Work out the finished part from the listing and answer in its coordinate system (mm). A direction names the side the tool comes from. Coordinates: 2 decimals unless noted, no trailing zeros. Write each loop counter-clockwise with the first axis right and the second up, starting at its lowest first coordinate (ties: lowest second). Pieces come first, ordered by that corner, then holes. Notation, with made-up numbers: (-23, 28.5) - (-16, 28.5) arc R20 ccw to (-16, 64.5) - close; hole circle Ø11 at (-4.75, 70). An arc over 180 degrees is marked (long way). Use a Markdown table: item, result. Add a question column.
(1) Given pin 1 Ø3 at (x, y) = (-41, 30) entering from +Z; pin 2 Ø5 at (x, z) = (-51.5, -6) entering from -Y; pin 3 Ø17 at (x, y) = (-66, 11.5) entering from +Z, each flat-ended and moving along its own axis, determine where each tip first touches the part or whether it passes through.
(2) For a pull along X with two mould halves and no side action, classify faces 5 (the face through (-78, 62, -127)), 6 (the face through (1, 0, 1)), 7 (the face through (54.98, 46.16, -63.82)) as released by +X, released by -X, zero draft, split by the parting line, or undercut.
(3) The part is cut by section A-A, the plane y = 49.5. Give the vertices of the cut face in (x, z), then the cut area to 3 significant figures.
(4) The part is cut by section C-C, the plane z = 97.5. Give the vertices of the cut face in (x, y), then the cut area to 3 significant figures.
(5) The part is cut by section B-B, the plane y = 70.5. Give the vertices of the cut face in (x, z), then the cut area to 4 significant figures.
(6) Find the intervals of material crossed by line 1 (X direction, y = 47, z = 97); line 2 (Z direction, x = 20.5, y = 42); line 3 (Z direction, x = -20, y = 42.5), in increasing order. Write a range as from..to.
(7) A tool of negligible diameter and unlimited length cuts with its end or side. For faces 1 (the face through (-68, 20, -47.5)), 2 (the face through (-29.53, 19.76, 50.84)), 3 (the face through (54.98, 46.16, 131.18)), 4 (the face through (29.041, 19.762, 51.032)), from which of +Z, -Z, +X, -X, +Y, -Y can it reach the whole face along a straight path? Write none if from no direction.
(8) The part is cut by section D-D, the plane x = 56.5. Give the vertices of the cut face in (y, z), then the cut area to 3 significant figures.
Autodesk Inventor part; units mm, degrees
ref_plane "YZ Plane" through (0, 0, 0) normal (1, 0, 0) x (0, 1, 0)
ref_plane "XZ Plane" through (0, 0, 0) normal (0, 1, 0) x (-1, 0, 0)
ref_plane "XY Plane" through (0, 0, 0) normal (0, 0, 1) x (1, 0, 0)
sketch "Sketch1" plane through (0, 0, 0) normal (0, 1, 0) x (-1, 0, 0)
  line L0 (-90, -140) -> (90, -140)
  line L1 (90, -140) -> (90, 140)
  line L2 (90, 140) -> (-90, 140)
  line L3 (-90, 140) -> (-90, -140)
  line L4 (-90, -140) -> (90, 140) construction
  line L5 (90, -140) -> (-90, 140) construction
  point P0 (0, 0)
  dimension "d0" = 280
  dimension "d1" = 180
extrude "Extrusion1" add sketch "Sketch1" along normal blind 80
sketch "Sketch2" plane through (0, 0, 0) normal (0, -1, 0) x (1, 0, 0)
  arc A0 (-47.5, 47.5) -> (2.5, 97.5) centre (-47.5, 97.5) ccw
  line L0 (0, 150) -> (0, -153.5615) construction
  line L1 (-95.9498, 0) -> (75.0535, 0) construction
  line L2 (2.5, 97.5) -> (2.5, 140)
  line L3 (-90, 47.5) -> (-47.5, 47.5)
  line L4 (-90, -140) -> (-90, 140)
  line L5 (-90, 47.5) -> (-90, 140)
  line L6 (-90, 140) -> (90, 140)
  line L7 (2.5, 140) -> (-90, 140)
  arc A1 (-2.5, 97.5) -> (47.5, 47.5) centre (47.5, 97.5) ccw
  line L8 (-2.5, 97.5) -> (-2.5, 140)
  line L9 (90, 47.5) -> (47.5, 47.5)
  line L10 (90, -140) -> (90, 140)
  line L11 (90, 140) -> (-90, 140)
  arc A2 (2.5, -97.5) -> (-47.5, -47.5) centre (-47.5, -97.5) ccw
  line L12 (2.5, -97.5) -> (2.5, -140)
  line L13 (-90, -47.5) -> (-47.5, -47.5)
  line L14 (-90, 140) -> (-90, -140)
  line L15 (-90, -140) -> (90, -140)
  line L16 (90, 140) -> (90, -140)
  line L17 (90, -47.5) -> (47.5, -47.5)
  arc A3 (47.5, -47.5) -> (-2.5, -97.5) centre (47.5, -97.5) ccw
  line L18 (-2.5, -97.5) -> (-2.5, -140)
  circle A4 centre (-47.5, 97.5) radius 34.5
  circle A5 centre (-47.5, 97.5) radius 42 construction
  line L19 (-89.5, 97.5) -> (-5.5, 97.5) construction
  line L20 (-47.5, 139.5) -> (-47.5, 55.5) construction
  line L21 (-77.1985, 127.1985) -> (-17.8015, 67.8015) construction
  line L22 (-17.8015, 127.1985) -> (-77.1985, 67.8015) construction
  point P0 (0, 0)
  point P1 (-2.5, -140)
  point P2 (90, -47.5)
  point P3 (-90, -47.5)
  point P4 (-2.5, 140)
  point P5 (75, -50)
  point P6 (-75, -50)
  dimension "d15" = 84
  dimension "d7" = 90
  dimension "d11" = 50
  dimension "d14" = 69
  dimension "d16" = 45
  dimension "d17" = 45
  dimension "d35" = 42.5
  dimension "d36" = 42.5
extrude "Extrusion2" cut sketch "Sketch2" against normal blind 40 contours L3 L4 L6 L8 A1 A0 | A1 L8 L6 L2 A0 | A0 L2 L6 L10 L9 A1 | L13 A2 A3 L18 L15 L4 | L10 L15 L12 A2 A3 L17 | L18 A3 A2 L12 L15 | A4
extrude "Extrusion3" cut sketch "Sketch2" against normal blind 12.5 from surface at -40 contours A4
mirror "Mirror1" about plane through (0, 0, 0) normal (0, 0, 1) of "Extrusion3"
mirror "Mirror2" about plane through (0, 0, 0) normal (1, 0, 0) of "Extrusion3", "Mirror1"
chamfer "Chamfer1" distance 25 angle 45 4 edges at (90, 60, 140) (-90, 60, 140) (90, 60, -140) (-90, 60, -140)
fillet "Fillet1" radius 20 2 edges at (0, 20, 81.8875) (0, 20, -81.8875)
chamfer "Chamfer2" distance 3 angle 45 26 edges at (0, 40, -140) (77.5, 40, -127.5) (90, 40, -81.25) (-77.5, 40, -127.5) (-90, 40, -81.25) (90, 40, 81.25) (77.5, 40, 127.5) (0, 40, 140) (-77.5, 40, 127.5) (-90, 40, 81.25) (-90, 0, 0) (-90, 20, 47.5) (-90, 20, -47.5) (-68.75, 0, -47.5) (-29.2837, 0, -50.9364) (0, 0, -66.0826) (29.2837, 0, -50.9364) (68.75, 0, -47.5) (-68.75, 0, 47.5) (-29.2837, 0, 50.9364) (0, 0, 66.0826) (29.2837, 0, 50.9364) (68.75, 0, 47.5) (90, 0, 0) (90, 20, -47.5) (90, 20, 47.5)
fillet "Fillet2" radius 3 8 edges at (29.2837, 40, -50.9364) (-29.2837, 40, -50.9364) (-67.25, 40, -47.5) (67.25, 40, -47.5) (29.2837, 40, 50.9364) (-29.2837, 40, 50.9364) (-67.25, 40, 47.5) (67.25, 40, 47.5)
chamfer "Chamfer4" distance 5 angle 45 2 edges at (90, 80, 0) (-90, 80, 0)
Model answer:
| question | item | result |
|---|---|---|
| 1 | pin 1 | z = 48.14 |
| 1 | pin 2 | y = 0 |
| 1 | pin 3 | z = 47.5 |
| 2 | face 5 | released by -X |
| 2 | face 6 | zero draft |
| 2 | face 7 | undercut |
| 3 | outline | (-90, -115) - (-65, -140) - (65, -140) - (90, -115) - (90, 115) - (65, 140) - (-65, 140) - (-90, 115) - close; hole circle Ø69 at (-47.5, -97.5); hole circle Ø69 at (-47.5, 97.5); hole circle Ø69 at (47.5, -97.5); hole circle Ø69 at (47.5, 97.5) |
| 3 | area | 34,200 mm^2 |
| 4 | outline | (-90, 43) - (-87, 40) - (-82, 40) - (-82, 52.5) - (-13, 52.5) - (-13, 40) - (13, 40) - (13, 52.5) - (82, 52.5) - (82, 40) - (87, 40) - (90, 43) - (90, 75) - (85, 80) - (-85, 80) - (-90, 75) - close |
| 4 | area | 5,440 mm^2 |
| 5 | outline | (-90, -115) - (-65, -140) - (65, -140) - (90, -115) - (90, 115) - (65, 140) - (-65, 140) - (-90, 115) - close |
| 5 | area | 49,150 mm^2 |
| 6 | line 1 | -90..-82, -13..13, 82..90 |
| 6 | line 2 | -139..-118.98, -76.02..76.02, 118.98..139 |
| 6 | line 3 | -139.5..-118.33, -76.67..76.67, 118.33..139.5 |
| 7 | face 1 | -Z, -X, -Y |
| 7 | face 2 | +Z, -X, -Y |
| 7 | face 3 | -Y |
| 7 | face 4 | +Z, +X, -Y |
| 8 | outline | (0, -44.5) - (3, -47.5) - (37, -47.5) arc R3 cw to (40, -50.5) - (40, -64.19) - (52.5, -64.19) - (52.5, -130.81) - (40, -130.81) - (40, -137) - (43, -140) - (80, -140) - (80, 140) - (43, 140) - (40, 137) - (40, 130.81) - (52.5, 130.81) - (52.5, 64.19) - (40, 64.19) - (40, 50.5) arc R3 cw to (37, 47.5) - (3, 47.5) - (0, 44.5) - close |
| 8 | area | 13,300 mm^2 |
